The model under review builds one solid part; all positions refer to its coordinate system, in mm. Face numbers are marked on the shaded views. Give positions to 0.01 mm unless a question says otherwise; leave off trailing zeros. Loops run counter-clockwise (first coordinate to the right, second up) from the corner with the lowest first, then second, coordinate; pieces in that order, holes last. Notation, with made-up numbers: M 16.5,77 L 58.5,77 A19 ccw 58.5,92 Z; hole C 34.25,20.25 d7. An arc over 180 degrees is marked long. Return JSON: item names as keys, results as strings.
Autodesk Inventor part; units mm, degrees
ref_plane "YZ Plane" through (0, 0, 0) normal (1, 0, 0) x (0, 1, 0)
ref_plane "XZ Plane" through (0, 0, 0) normal (0, 1, 0) x (-1, 0, 0)
ref_plane "XY Plane" through (0, 0, 0) normal (0, 0, 1) x (1, 0, 0)
sketch "Sketch1" plane through (0, 0, 0) normal (0, 0, 1) x (1, 0, 0)
  line L0 (75, 0) -> (75, 27)
  line L1 (75, 27) -> (0, 27)
  line L2 (0, 27) -> (0, 0)
  line L3 (31.5, 0) -> (31.5, 13.5)
  arc A0 (43.5, 13.5) -> (31.5, 13.5) centre (37.5, 13.5) ccw
  line L4 (43.5, 13.5) -> (43.5, 0)
  line L5 (0, 0) -> (31.5, 0)
  line L6 (43.5, 0) -> (75, 0)
  circle A1 centre (12.5, 13.5) radius 2.1
  circle A2 centre (62.5, 13.5) radius 2.1
  point P0 (37.5, 27)
  point P1 (0, 13.5)
  dimension "d0" = 12
  dimension "d1" = 4.2
  dimension "d2" = 50
  dimension "d3" = 25
  dimension "d4" = 75
  dimension "d6" = 13.5
extrude "Extrusion1" add sketch "Sketch1" along normal blind 4.6
chamfer "Chamfer1" distance 4 angle 45 4 edges at (0, 27, 2.3) (0, 0, 2.3) (75, 0, 2.3) (75, 27, 2.3)
chamfer "Chamfer2" distance 2 angle 45 2 edges at (31.5, 0, 2.3) (43.5, 0, 2.3)
chamfer "Chamfer3" distance 1 angle 45 4 edges at (10.4, 13.5, 4.6) (10.4, 13.5, 0) (60.4, 13.5, 0) (60.4, 13.5, 4.6)
equation "\"d3\" = 0.5 * d2"
properties part number "hotend_mount" material "Polycarbonate, Clear"
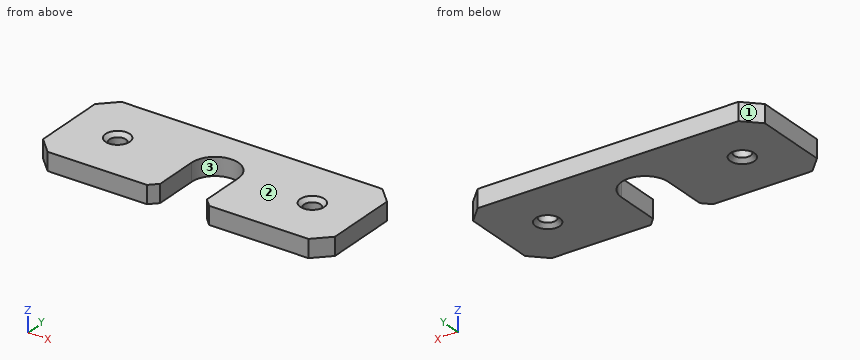
1) Insertion check: pin 1 (5.5 mm diameter, centred on x = 62.5, y = 13.5, fed in from +Z). The pin has a flat end and moves straight along its axis. Give the tip position at first contact, or say it passes through.
From the geometry:
{"pin 1": "z = 4.25"}
2) Consider section B-B on x = 37.5. Write out the cut boundary in (y, z), then the cut area to 3 significant figures.
From the geometry:
{"outline": "M 19.5,0 L 27,0 L 27,4.6 L 19.5,4.6 Z", "area": "34.5 mm²"}
3) Consider section C-C on y = 25. Write out the cut boundary in (x, z), then the cut area to 3 significant figures.
From the geometry:
{"outline": "M 2,0 L 73,0 L 73,4.6 L 2,4.6 Z", "area": "327 mm²"}
4) Consider section A-A on x = 12.5. Write out the cut boundary in (y, z), then the cut area to 3 significant figures.
From the geometry:
{"outline": "M 0,0 L 10.4,0 L 11.4,1 L 11.4,3.6 L 10.4,4.6 L 0,4.6 Z; M 15.6,1 L 16.6,0 L 27,0 L 27,4.6 L 16.6,4.6 L 15.6,3.6 Z", "area": "103 mm²"}
5) Wall thickness on L1, parallel to X at y = 13, z = 1.65; L2, parallel to X at y = 5.75, z = 3.35; L3, parallel to Y at x = 62.5, z = 2.1: over which ranges is each line inside the solid? List them lowest first. Write a range as from..to.
From the geometry:
{"L1": "0..10.46, 14.54..31.5, 43.5..60.46, 64.54..75", "L2": "0..31.5, 43.5..75", "L3": "0..11.4, 15.6..27"}
6) The part is to be moulded in two halves that separate along X. For the marked faces 1, 2 and 3, say which applies: released by +X, released by -X, zero draft, split by the parting line, or undercut.
From the geometry:
{"face 1": "released by -X", "face 2": "zero draft", "face 3": "undercut"}
